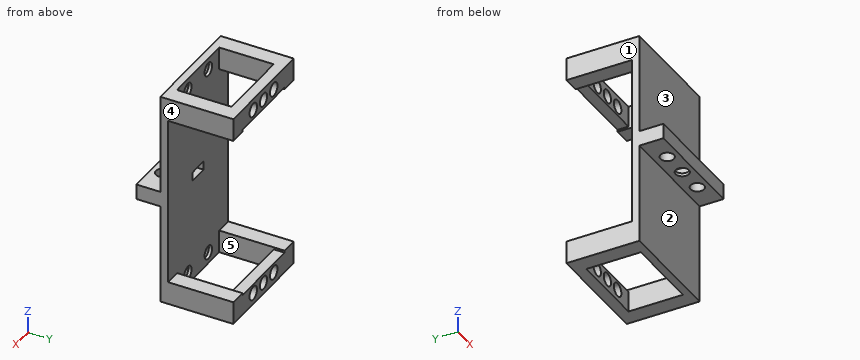
Autodesk Inventor part; units mm, degrees
ref_plane "YZ Plane" through (0, 0, 0) normal (1, 0, 0) x (0, 1, 0)
ref_plane "XZ Plane" through (0, 0, 0) normal (0, 1, 0) x (-1, 0, 0)
ref_plane "XY Plane" through (0, 0, 0) normal (0, 0, 1) x (1, 0, 0)
sketch "Skizze1" plane through (0, 0, 0) normal (0, 0, 1) x (1, 0, 0)
  line L0 (-6.5297, -2.8796) -> (43.4703, -2.8796)
  line L1 (43.4703, -2.8796) -> (43.4703, 8.1204)
  line L2 (43.4703, 8.1204) -> (-6.5297, 8.1204)
  line L3 (-6.5297, 8.1204) -> (-6.5297, -2.8796)
  point P0 (0, 0)
  dimension "d0" = 50
  dimension "d1" = 11
extrude "Extrusion1" add sketch "Skizze1" along normal blind 7
sketch "Skizze2" plane through (-6.5297, 8.1204, 0) normal (0, 1, 0) x (1, 0, 0)
  line L0 (29.65, -5.55) -> (20.35, -5.55)
  line L1 (20.35, -5.55) -> (20.35, -1.45)
  line L2 (20.35, -1.45) -> (29.65, -1.45)
  line L3 (29.65, -1.45) -> (29.65, -5.55)
  line L4 (50, -7) -> (0, -7)
  line L5 (50, 0) -> (50, -7)
  line L6 (0, 0) -> (0, -7)
  point P0 (6.5297, 0)
  dimension "d4" = 9.3
  dimension "d5" = 4.1
  dimension "d6" = 1.45
  dimension "d7" = 20.35
  dimension "d8" = 20.35
extrude "Extrusion2" cut sketch "Skizze2" against normal blind 9.35
sketch "Skizze3" plane through (0, 0, 7) normal (0, 0, 1) x (1, 0, 0)
  line L0 (-6.5297, 8.1204) -> (-6.5297, -2.8796)
  line L1 (43.4703, 8.1204) -> (-6.5297, 8.1204)
  point P0 (0, 0)
  point P1 (5.9703, 2.2704)
  point P2 (18.4703, 2.2704)
  point P3 (30.9703, 2.2704)
  dimension "d11" = 12.5
  dimension "d12" = 12.5
  dimension "d13" = 12.5
  dimension "d14" = 5.85
hole "Bohrung1" at (5.9703, 2.2704, 7) at (18.4703, 2.2704, 7) at (30.9703, 2.2704, 7) direction (0, 0, -1) diameter 6.15 end through all
sketch "Skizze4" plane through (-6.5297, 8.1204, 0) normal (0, 1, 0) x (1, 0, 0)
  point P0 (6.5297, 0)
sketch "Skizze5" plane through (-6.5297, 8.1204, 0) normal (0, 1, 0) x (1, 0, 0)
  line L0 (50, 0) -> (0, 0)
  line L1 (0, 0) -> (0, -53.0037)
  line L2 (0, -53) -> (50, -53)
  line L3 (50, -53) -> (50, 46)
  line L4 (50, 46) -> (0, 46)
  line L5 (0, 46) -> (0, -53)
  point P0 (6.5297, 0)
  dimension "d22" = 50
  dimension "d23" = 99
  dimension "d24" = 46
extrude "Extrusion3" add sketch "Skizze5" along normal blind 3.5
sketch "Skizze6" plane through (-6.5297, 11.6204, 0) normal (0, 1, 0) x (1, 0, 0)
  line L0 (29.65, -1.45) -> (29.65, -5.55)
  line L1 (29.65, -1.45) -> (20.35, -1.45)
  line L2 (20.35, -1.45) -> (20.35, -5.55)
  line L3 (20.35, -5.55) -> (29.65, -5.55)
  line L4 (29.65, -5.55) -> (29.65, -1.45)
  point P0 (6.5297, 0)
extrude "Extrusion4" cut sketch "Skizze6" against normal blind 3.5
sketch "Skizze7" plane through (-6.5297, 11.6204, 0) normal (0, 1, 0) x (1, 0, 0)
  line L0 (0, -53) -> (50, -53)
  line L1 (50, -53) -> (42.5, -53)
  line L2 (42.5, -53) -> (42.5, -42.5)
  line L3 (42.5, -42.5) -> (50, -42.5)
  line L4 (50, -42.5) -> (50, -53)
  line L5 (0, -53) -> (7.5, -53)
  line L6 (7.5, -53) -> (7.5, -42.5)
  line L7 (7.5, -42.5) -> (0, -42.5)
  line L8 (0, -42.5) -> (0, -53)
  line L9 (0, 46) -> (0, -53)
  line L10 (0, 46) -> (7.5, 46)
  line L11 (7.5, 46) -> (7.5, 35.5)
  line L12 (7.5, 35.5) -> (0, 35.5)
  line L13 (0, 35.5) -> (0, 46)
  line L14 (50, -53) -> (50, 46)
  line L15 (50, 46) -> (42.5, 46)
  line L16 (42.5, 46) -> (42.5, 35.5)
  line L17 (42.5, 35.5) -> (50, 35.5)
  line L18 (50, 35.5) -> (50, 46)
  point P0 (6.5297, 0)
  dimension "d29" = 7.5
  dimension "d30" = 10.5
  dimension "d31" = 7.5
  dimension "d32" = 10.5
  dimension "d33" = 7.5
  dimension "d34" = 10.5
  dimension "d35" = 7.5
  dimension "d36" = 10.5
extrude "Extrusion5" add sketch "Skizze7" along normal blind 25
sketch "Skizze8" plane through (0.9703, 11.6204, -35.5) normal (1, 0, 0) x (0, 0, -1)
  point P0 (-35.5, -11.6204)
sketch "Skizze9" plane through (-6.5297, 36.6204, 0) normal (0, 1, 0) x (1, 0, 0)
  line L0 (50, -42.5) -> (50, 35.5)
  line L1 (0, 46) -> (50, 46)
  line L2 (50, 46) -> (50, 35.5)
  line L3 (50, 35.5) -> (0, 35.5)
  line L4 (0, 35.5) -> (0, 46)
  line L5 (50, -53) -> (50, -7)
  line L6 (0, -42.5) -> (50, -42.5)
  line L7 (50, -42.5) -> (50, -53)
  line L8 (50, -53) -> (0, -53)
  line L9 (0, -53) -> (0, -42.5)
  line L10 (50, -42.5) -> (42.5, -42.5)
  point P0 (6.5297, 0)
  dimension "d75" = 0
extrude "Extrusion6" add sketch "Skizze9" along normal blind 5
sketch "Skizze10" plane through (-6.5297, 41.6204, 0) normal (0, 1, 0) x (1, 0, 0)
  line L0 (50, 46) -> (0, 46)
  line L1 (0, -53) -> (50, -53)
  line L2 (42.5, -42.5) -> (42.5, -53)
  line L3 (42.5, 46) -> (42.5, 35.5)
  line L4 (7.5, 35.5) -> (7.5, 46)
  line L5 (7.5, -53) -> (7.5, -42.5)
  point P0 (6.5297, 0)
  point P1 (15.7518, 40.75)
  point P2 (25, 40.75)
  point P3 (33.5, 40.75)
  point P4 (15.6745, -47.75)
  point P5 (25, -47.75)
  point P6 (33.5, -47.75)
  dimension "d41" = 5.25
  dimension "d42" = 5.25
  dimension "d43" = 5.25
  dimension "d44" = 5.25
  dimension "d45" = 5.25
  dimension "d46" = 5.25
  dimension "d47" = 9
  dimension "d50" = 9
  dimension "d76" = 17.5
  dimension "d77" = 17.5
hole "Bohrung2" at (18.4703, 41.6204, 47.75) at (18.4703, 41.6204, -40.75) direction (0, -1, 0) diameter 6 depth 10 tip angle 118
sketch "Skizze11" plane through (-6.5297, 41.6204, 0) normal (0, 1, 0) x (1, 0, 0)
  line L0 (7.5, -53) -> (7.5, -42.5)
  line L1 (42.5, -42.5) -> (42.5, -53)
  line L2 (50, -42.5) -> (0, -42.5)
  line L3 (50, 46) -> (0, 46)
  line L4 (42.5, 46) -> (42.5, 35.5)
  line L5 (7.5, 35.5) -> (7.5, 46)
  point P0 (6.5297, 0)
  point P1 (16.5, -47.75)
  point P2 (33.5, -47.75)
  point P3 (16.5, 40.75)
  point P4 (33.5, 40.75)
  dimension "d60" = 9
  dimension "d61" = 9
  dimension "d62" = 5.25
  dimension "d63" = 5.25
  dimension "d64" = 5.25
  dimension "d65" = 5.25
  dimension "d66" = 9
  dimension "d67" = 9
hole "Bohrung3" at (9.9703, 41.6204, 47.75) at (26.9703, 41.6204, 47.75) at (9.9703, 41.6204, -40.75) at (26.9703, 41.6204, -40.75) direction (0, -1, 0) diameter 6.2 depth 31.5 tip angle 118
sketch "Skizze12" plane through (-6.5297, -2.8796, 0) normal (0, -1, 0) x (1, 0, 0)
  point P0 (6.5297, 0)
sketch "Skizze13" plane through (-6.5297, 41.6204, 0) normal (0, 1, 0) x (1, 0, 0)
  line L0 (42.5, -53) -> (42.5, -42.5)
  line L1 (7.5, -42.5) -> (7.5, -53)
  line L2 (42.5, -42.5) -> (7.5, -42.5)
  line L3 (7.5, -42.5) -> (7.5, -43.46)
  line L4 (7.5, -43.46) -> (42.5, -43.46)
  line L5 (42.5, -43.46) -> (42.5, -42.5)
  point P0 (6.5297, 0)
  dimension "d78" = 0.96
extrude "Extrusion7" cut sketch "Skizze13" against normal blind 10
sketch "Skizze14" plane through (35.9703, 11.6204, -35.5) normal (0, 0, 1) x (1, 0, 0)
  point P0 (-35.9703, -11.6204)
sketch "Skizze15" plane through (-6.5297, 41.6204, 0) normal (0, 1, 0) x (1, 0, 0)
  line L0 (7.5, 46) -> (7.5, 35.5)
  line L1 (42.5, 35.5) -> (7.5, 35.5)
  line L2 (7.5, 35.5) -> (7.5, 36.48)
  line L3 (7.5, 36.48) -> (42.5, 36.48)
  line L4 (42.5, 36.48) -> (42.5, 35.5)
  line L5 (0, 35.5) -> (50, 35.5)
  point P0 (6.5297, 0)
  dimension "d81" = 0.98
  dimension "d82" = 0
extrude "Extrusion8" cut sketch "Skizze15" against normal blind 10
properties part number "Objektträgerhalter 1.1 final"
Verification items for the finished model (mm, model axes). Face numbers are marked on the shaded views. A direction names the side the tool comes from. Give positions to 0.01 mm unless a question says otherwise; leave off trailing zeros. Loops run counter-clockwise (first coordinate to the right, second up) from the corner with the lowest first, then second, coordinate; pieces in that order, holes last.
1. Release check for a two-part mould opening along Y. For the marked faces 3, 4 and 5 record: +Y half, -Y half, draft (parallel to the pull), parting line (faces both ways), or undercut.
Derived:
face 3: -Y half
face 4: draft
face 5: undercut
2. Cross-section at B-B on x = 32. Record the cut outline in (y, z), and give its area (3 significant figures).
Derived:
outline: (-2.88, 0) - (-0.63, 0) - (-0.63, 7) - (-2.88, 7) - close; (5.17, 0) - (8.12, 0) - (8.12, -46) - (11.62, -46) - (11.62, 53) - (8.12, 53) - (8.12, 7) - (5.17, 7) - close; (36.62, -46) - (41.62, -46) - (41.62, -36.48) - (36.62, -36.48) - close; (36.62, 43.46) - (41.62, 43.46) - (41.62, 53) - (36.62, 53) - close
area: 478 mm2
3. Go/stop test with flat-tipped pins: P1, Ø10, axis at x = 34.5, y = 34.5, coming from the -Z side; P2, Ø5, axis at x = 18.47, y = 2.27, coming from the +Z side; P3, Ø10, axis at x = 26.97, z = -40.75, coming from the -Y side; P4, Ø3.5, axis at x = 21, y = 1.5, coming from the +Z side. Record where each tip stops, or that it passes through.
Derived:
P1: stops at z = -46
P2: passes through
P3: stops at y = 8.12
P4: stops at z = 7
4. Tool access check on the marked faces 1 and 2. Record the directions out of +Z, -Z, +X, -X, +Y, -Y that give a thin tool (end or side, any length) a straight path to the whole face; none if there is none.
Derived:
face 1: +Z, -Z, -X, +Y, -Y
face 2: -Z, +X, -X, -Y
5. Cross-section at A-A on y = 39. Record the cut outline in (x, z), and give its area (3 significant figures).
Derived:
outline: (-6.53, -46) - (43.47, -46) - (43.47, -35.5) - (35.97, -35.5) - (35.97, -36.48) - (0.97, -36.48) - (0.97, -35.5) - (-6.53, -35.5) - close; (-6.53, 42.5) - (0.97, 42.5) - (0.97, 43.46) - (35.97, 43.46) - (35.97, 42.5) - (43.47, 42.5) - (43.47, 53) - (-6.53, 53) - close; hole circle Ø6.2 at (9.97, -40.75); hole circle Ø6.2 at (9.97, 47.75); hole circle Ø6 at (18.47, -40.75); hole circle Ø6 at (18.47, 47.75); hole circle Ø6.2 at (26.97, -40.75); hole circle Ø6.2 at (26.97, 47.75)
area: 805 mm2
6. Material ranges on probe 1 along X at (y, z) = (38.6, -40.75); probe 2 along X at (y, z) = (10.85, -40.75); probe 3 along X at (y, z) = (23, 48), recorded low to high.
Derived:
probe 1: x = -6.53 to 6.87, 13.07 to 15.47, 21.47 to 23.87, 30.07 to 43.47
probe 2: x = -6.53 to 6.87, 13.07 to 23.87, 30.07 to 43.47
probe 3: x = -6.53 to 0.97, 35.97 to 43.47
7. Cross-section at C-C on y = 6.5. Record the cut outline in (x, z), and give its area (3 significant figures).
Derived:
outline: (-6.53, 0) - (43.47, 0) - (43.47, 7) - (-6.53, 7) - close; hole (13.82, 1.45) - (23.12, 1.45) - (23.12, 5.55) - (13.82, 5.55) - close
area: 312 mm2
8. Cross-section at D-D on z = -24. Record the cut outline in (x, y).
Derived:
outline: (-6.53, 8.12) - (43.47, 8.12) - (43.47, 11.62) - (-6.53, 11.62) - close
